from build123d import *

# Parameters (mm, degrees)
SALIENTE_EXTRUIR1_DEPTH = 3
SALIENTE_EXTRUIR2_DEPTH = 30


with BuildPart() as part:
    # Croquis1 → Saliente-Extruir1 (new body)
    with BuildSketch(Plane(origin=(0, 0, 0), x_dir=(1, 0, 0), z_dir=(0, 1, 0))):
        Polygon((50, 20), (150, 20), (150, 30), (200, 30), (200, 175), (0, 175), (0, 30), (50, 30), align=None)
    extrude(amount=SALIENTE_EXTRUIR1_DEPTH)

    # Croquis2 → Saliente-Extruir2 (add)
    with BuildSketch(Plane(origin=(0, 3, 0), x_dir=(1, 0, 0), z_dir=(0, 1, 0))):
        Polygon((0, 175), (200, 175), (200, 30), (150, 30), (150, 20), (50, 20), (50, 30), (0, 30), align=None)
        Polygon((197, 33), (197, 172), (3, 172), (3, 33), (53, 33), (53, 23), (147, 23), (147, 33), align=None, mode=Mode.SUBTRACT)
    extrude(amount=SALIENTE_EXTRUIR2_DEPTH)


solid = part.part
CAD build for the part. Positions are in the model's coordinates, mm. A direction names the side the tool comes from. Coordinates: 2 decimals unless noted, no trailing zeros. Order: outer loops, then holes, each group sorted by start corner. A loop starts at its lowest first (then second) coordinate and runs counter-clockwise, first axis right, second up.
Item 1: Two-plate mould, pull along Z, no slides. Class faces 6 (the face through (175, 16, -30)), 7 (the face through (100.5, 33, -172.5)), 8 (the face through (99, 18, -23)): +Z half, -Z half, draft (parallel to the pull), parting line (faces both ways), or undercut.
Check sheet entries:
face 6: +Z half
face 7: draft
face 8: undercut
Item 2: Band-saw the part on B-B on x = 86.5. List the corners of the cut face in (y, z).
Check sheet entries:
outline: (0, -175) - (33, -175) - (33, -172) - (3, -172) - (3, -23) - (33, -23) - (33, -20) - (0, -20) - close
Item 3: Band-saw the part on A-A on y = 24. List the corners of the cut face in (x, z).
Check sheet entries:
outline: (0, -175) - (200, -175) - (200, -30) - (150, -30) - (150, -20) - (50, -20) - (50, -30) - (0, -30) - close; hole (3, -172) - (197, -172) - (197, -33) - (147, -33) - (147, -23) - (53, -23) - (53, -33) - (3, -33) - close
Item 4: Drill centre lines: L1, parallel to X at y = 11, z = -163; L2, parallel to Z at x = 179.5, y = 12; L3, parallel to Z at x = 89.5, y = 6. Where is each one in solid material? Low to high.
Check sheet entries:
L1: x = 0 to 3, 197 to 200
L2: z = -175 to -172, -33 to -30
L3: z = -175 to -172, -23 to -20
Item 5: 3-axis set-ups, long thin cutter, end or side, ignore diameter. For faces 1 (the face through (25, 16, -30)), 2 (the face through (150, 16, -25)), 3 (the face through (200, 16, -104)), 4 (the face through (3, 18, -103)), 5 (the face through (0, 16, -101)): which of +Z, -Z, +X, -X, +Y, -Y reach the whole face in a straight line?
Check sheet entries:
face 1: +Z, -X, +Y, -Y
face 2: +Z, +X, +Y, -Y
face 3: +Z, -Z, +X, +Y, -Y
face 4: +Y
face 5: +Z, -Z, -X, +Y, -Y
Item 6: Pin check, flat tips, straight feed: pin 1 Ø8 at (y, z) = (19, -23.5) entering from +X; pin 2 Ø4 at (x, z) = (153.5, -88.5) entering from +Y; pin 3 Ø16.5 at (x, y) = (167, 9) entering from +Z. Stop position of each tip, or through.
Check sheet entries:
pin 1: stops at x = 150
pin 2: stops at y = 3
pin 3: stops at z = -30
Item 7: Band-saw the part on C-C on z = -160.5. List the corners of the cut face in (x, y).
Check sheet entries:
outline: (0, 0) - (200, 0) - (200, 33) - (197, 33) - (197, 3) - (3, 3) - (3, 33) - (0, 33) - close
